from build123d import *

# Parameters (mm, degrees)
EXTRUDE_1_DEPTH      = 43
SKETCH_2_R           = 1.5
EXTRUDE_2_DEPTH      = 6
CHAMFER_1_SIZE       = 0.2
SKETCH_3_R           = 1.229375
CUT_EXTRUDE_1_DEPTH  = 6
SKETCH_4_OUTSIDE_W   = 26.892
SKETCH_4_OUTSIDE_H   = 27.604
SKETCH_4_OUTSIDE_R   = 2.3
CUT_EXTRUDE_2_DEPTH  = 3
CUT_EXTRUDE_2_DRAFT  = -60
CUT_EXTRUDE_START    = -43
SKETCH_4_2_OUTSIDE_W = 26.892
SKETCH_4_2_OUTSIDE_H = 27.604
SKETCH_4_2_OUTSIDE_R = 2.3
CUT_EXTRUDE_3_DEPTH  = 3
CUT_EXTRUDE_3_DRAFT  = 60
CHAMFER_2_SIZE       = 0.2


with BuildPart() as part:
    # 草图1 → 凸台-拉伸1 (new body)
    with BuildSketch(Plane(origin=(0, 0, 0), x_dir=(1, 0, 0), z_dir=(0, 1, 0))):
        Polygon((0, 2.655811238), (-2.3, 1.327905619), (-2.3, -1.327905619), (0, -2.655811238), (2.3, -1.327905619), (2.3, 1.327905619), align=None)
    extrude(amount=EXTRUDE_1_DEPTH)

    # 草图2 → 凸台-拉伸2 (add)
    with BuildSketch(Plane(origin=(0, 43, 0), x_dir=(1, 0, 0), z_dir=(0, 1, 0))):
        with Locations(Location((0, 0, 0), (0, 0, 270))):
            Circle(SKETCH_2_R)
    extrude(amount=EXTRUDE_2_DEPTH)

    # 倒角1
    chamfer_1_edges = [part.edges().sort_by_distance(p)[0] for p in [
        (0, 49, -1.5),
    ]]
    chamfer(chamfer_1_edges, length=CHAMFER_1_SIZE)

    # 草图3 → 切除-拉伸1 (cut)
    with BuildSketch(Plane.XZ):
        with Locations(Location((0, 0, 0), (0, 0, 270))):
            Circle(SKETCH_3_R)
    extrude(amount=-CUT_EXTRUDE_1_DEPTH, mode=Mode.SUBTRACT)


with BuildPart() as cut_extrude_2_tool:
    # 草图4 outside → 切除-拉伸2 (with draft: the straight prism first)
    with BuildSketch(Plane.XZ):
        Rectangle(SKETCH_4_OUTSIDE_W, SKETCH_4_OUTSIDE_H)
        Circle(SKETCH_4_OUTSIDE_R, mode=Mode.SUBTRACT)
    extrude(amount=-CUT_EXTRUDE_2_DEPTH)
    # 切除-拉伸2: the draft: its side faces are tilted about the plane it starts from
    cut_extrude_2_sides = [cut_extrude_2_tool.faces().sort_by_distance(p)[0] for p in [
        (0, 1.5, -13.802),
        (13.446, 1.5, 0),
        (0, 1.5, 13.802),
        (-13.446, 1.5, 0),
        (-2.3, 1.5, 0),
    ]]
    draft(cut_extrude_2_sides, Plane.XZ, CUT_EXTRUDE_2_DRAFT)


with BuildPart() as part_1:
    add(part.part)

    # 切除-拉伸2: cut by cut_extrude_2_tool
    add(cut_extrude_2_tool.part, mode=Mode.SUBTRACT)


with BuildPart() as cut_extrude_3_tool:
    # 草图4<2> outside → 切除-拉伸3 (with draft: the straight prism first)
    with BuildSketch(Plane.XZ.offset(CUT_EXTRUDE_START)):
        Rectangle(SKETCH_4_2_OUTSIDE_W, SKETCH_4_2_OUTSIDE_H)
        Circle(SKETCH_4_2_OUTSIDE_R, mode=Mode.SUBTRACT)
    extrude(amount=CUT_EXTRUDE_3_DEPTH)
    # 切除-拉伸3: the draft: its side faces are tilted about the plane it starts from
    cut_extrude_3_sides = [cut_extrude_3_tool.faces().sort_by_distance(p)[0] for p in [
        (0, 41.5, -13.802),
        (13.446, 41.5, 0),
        (0, 41.5, 13.802),
        (-13.446, 41.5, 0),
        (-2.3, 41.5, 0),
    ]]
    draft(cut_extrude_3_sides, Plane.XZ.offset(CUT_EXTRUDE_START), CUT_EXTRUDE_3_DRAFT)


with BuildPart() as part_2:
    add(part_1.part)

    # 切除-拉伸3: cut by cut_extrude_3_tool
    add(cut_extrude_3_tool.part, mode=Mode.SUBTRACT)

    # 倒角2
    chamfer_2_edges = [part_2.edges().sort_by_distance(p)[0] for p in [
        (0, 0, 1.229375),
    ]]
    chamfer(chamfer_2_edges, length=CHAMFER_2_SIZE)


solid = part_2.part
Input: part model. Units: mm. Frame: model coordinates. A direction names the side the tool comes from. Coordinates: 2 decimals unless noted, no trailing zeros. Order: outer loops, then holes, each group sorted by start corner. A loop starts at its lowest first (then second) coordinate and runs counter-clockwise, first axis right, second up.
1. Contact query for a flat-ended pin moving along its axis: P1, Ø1.2, axis at x = 0, z = -0.5, coming from the -Y side. Output: stop coordinate, or through.
Checked values:
P1: stops at y = 6
2. Access query for faces 4 (the flat face through (0, 43, 2)), 5 (the flat face through (-1.134, 21.199, -2.001)). Directions: +Z, -Z, +X, -X, +Y, -Y. A direction counts if a zero-diameter tool reaches every point of the face in a straight line with its end or side. Return the directions, or none.
Checked values:
face 4: +Y
face 5: -Z, -X, +Y, -Y
3. Cut plane A-A, the plane y = 4. Return loops of the section in (x, z).
Checked values:
outline: (-2.3, -1.33) - (0, -2.66) - (2.3, -1.33) - (2.3, 1.33) - (0, 2.66) - (-2.3, 1.33) - close; hole circle Ø2.46 at (0, 0)
4. Draft query along Z for faces 1 (the conical face through (2.13, 0.09, 1.22)), 2 (the cylindrical face through (1.22, 3.06, 0.16)), 3 (the conical face through (-2.13, 0.09, -1.22)). Return one class per face: +Z half, -Z half, draft (parallel to the pull), parting line (faces both ways), or undercut.
Checked values:
face 1: +Z half
face 2: undercut
face 3: -Z half
5. Cut plane B-B, the plane y = 29. Return loops of the section in (x, z), plus the area to 3 significant figures.
Checked values:
outline: (-2.3, -1.33) - (0, -2.66) - (2.3, -1.33) - (2.3, 1.33) - (0, 2.66) - (-2.3, 1.33) - close
area: 18.3 mm2
6. Ray query, line 1 along X through (y, z) = (4.4, 0); line 2 along Y through (x, z) = (0.45, 0.3); line 3 along Y through (x, z) = (1.55, -0.05). Return the intervals inside material, ascending.
Checked values:
line 1: x = -2.3 to -1.23, 1.23 to 2.3
line 2: y = 6 to 49
line 3: y = 0 to 43
